from build123d import *

# Parameters (mm, degrees)
ESQUISSE1_W             = 35.1
ESQUISSE1_H             = 55.9
ESQUISSE1_W_2           = 20.1
ESQUISSE1_H_2           = 40.9
BOSS_EXTRU_1_DEPTH      = 4
ESQUISSE5_W             = 17.55
ESQUISSE5_H             = 3
BOSS_EXTRU_2_DEPTH      = 4
ESQUISSE7_W             = 11.4
ESQUISSE7_H             = 7
BOSS_EXTRU_3_DEPTH      = 6
ESQUISSE8_R             = 3
ENL_V_MAT_EXTRU_1_DEPTH = 6
CONG_1_R                = 0.5
CONG_2_R                = 0.5
ENL_V_MAT_EXTRU_2_REACH = 47.983
ESQUISSE9_R             = 2.25


with BuildPart() as part:
    # Esquisse1 → Boss.-Extru.1 (new body)
    with BuildSketch(Plane(origin=(0, 0, 0), x_dir=(1, 0, 0), z_dir=(0, 1, 0))):
        with Locations((-6.45, -0.55)):
            Rectangle(ESQUISSE1_W, ESQUISSE1_H)
        with Locations((-6.45, -0.55)):
            Rectangle(ESQUISSE1_W_2, ESQUISSE1_H_2, mode=Mode.SUBTRACT)
    extrude(amount=BOSS_EXTRU_1_DEPTH)

    # Esquisse5 → Boss.-Extru.2 (add)
    with BuildSketch(Plane.XY.offset(28.5)):
        with Locations((2.325, 5.5)):
            Rectangle(ESQUISSE5_W, ESQUISSE5_H)
    boss_extru_2 = extrude(amount=-BOSS_EXTRU_2_DEPTH)

    # Symétrie1: Boss.-Extru.2 across plane
    add(boss_extru_2.mirror(Plane(origin=(-6.45, 0, 0), x_dir=(0, 0, 1), z_dir=(1, 0, 0))))

    # Esquisse7 → Boss.-Extru.3 (add)
    with BuildSketch(Plane.XY.offset(28.5)):
        with Locations((16.8, 3.5)):
            Rectangle(ESQUISSE7_W, ESQUISSE7_H)
    boss_extru_3 = extrude(amount=-BOSS_EXTRU_3_DEPTH)

    # Esquisse8 → Enlèv. mat.-Extru.1 (cut)
    with BuildSketch(Plane(origin=(0, 0, 22.5), x_dir=(-1, 0, 0), z_dir=(0, 0, -1))):
        with Locations((-16.8, 3.5)):
            Circle(ESQUISSE8_R)
    enl_v_mat_extru_1 = extrude(amount=-ENL_V_MAT_EXTRU_1_DEPTH, mode=Mode.SUBTRACT)

    # Symétrie2: Boss.-Extru.3 across plane
    add(boss_extru_3.mirror(Plane(origin=(-6.45, 0, 0), x_dir=(0, 0, 1), z_dir=(1, 0, 0))))

    # Symétrie3: Enlèv. mat.-Extru.1 across plane
    add(enl_v_mat_extru_1.mirror(Plane(origin=(-6.45, 0, 0), x_dir=(0, 0, 1), z_dir=(1, 0, 0))), mode=Mode.SUBTRACT)

    # Congé1
    cong_1_edges = [part.edges().sort_by_distance(p)[0] for p in [
        (11.1, 7, 23.5),
        (-24, 7, 23.5),
        (-24, 0, -2.45),
        (11.1, 0, -2.45),
        (11.1, 5.5, 24.5),
        (-6.45, 7, 24.5),
        (-24, 5.5, 24.5),
        (-6.45, 4, 24.5),
        (-29.7, 7, 22.5),
        (-35.4, 3.5, 22.5),
        (-29.7, 0, 22.5),
        (-24, 2, 22.5),
        (11.1, 2, 22.5),
        (16.8, 0, 22.5),
        (22.5, 3.5, 22.5),
        (16.8, 7, 22.5),
    ]]
    fillet(cong_1_edges, radius=CONG_1_R - 0.0001)  # a hair under: the kernel refuses the full size

    # Congé2
    cong_2_edges = [part.edges().sort_by_distance(p)[0] for p in [
        (-6.45, 0, -27.4),
        (10.95358268, 0.14641732, -27.4),
        (-23.85358268, 0.14641732, -27.4),
        (-6.45, 4, -27.4),
        (11.1, 2.24995, -27.4),
        (-24, 2.24995, -27.4),
    ]]
    fillet(cong_2_edges, radius=CONG_2_R - 0.0001)  # a hair under: the kernel refuses the full size

    # Esquisse9 → Enlèv. mat.-Extru.2 (cut, up to next)
    with BuildSketch(Plane.XZ, mode=Mode.PRIVATE) as enl_v_mat_extru_2_sk1:
        with Locations(Location((-1.95, -24.9, 0), (0, 0, 297.266044451))):
            Circle(ESQUISSE9_R)
    enl_v_mat_extru_2_tool1 = extrude(enl_v_mat_extru_2_sk1.sketch, amount=-ENL_V_MAT_EXTRU_2_REACH, mode=Mode.PRIVATE) & part.part
    # Esquisse9 → Enlèv. mat.-Extru.2 (cut, up to next)
    with BuildSketch(Plane.XZ, mode=Mode.PRIVATE) as enl_v_mat_extru_2_sk2:
        with Locations(Location((-10.95, -24.9, 0), (0, 0, 242.733955549))):
            Circle(ESQUISSE9_R)
    enl_v_mat_extru_2_tool2 = extrude(enl_v_mat_extru_2_sk2.sketch, amount=-ENL_V_MAT_EXTRU_2_REACH, mode=Mode.PRIVATE) & part.part
    add(enl_v_mat_extru_2_tool1.solids().sort_by_distance((-1.95, 0, -24.9))[0], mode=Mode.SUBTRACT)
    add(enl_v_mat_extru_2_tool2.solids().sort_by_distance((-10.95, 0, -24.9))[0], mode=Mode.SUBTRACT)


solid = part.part
Geometry check sheet. Reference: the model listing, model coordinates, mm. A direction names the side the tool comes from. Give positions to 0.01 mm unless a question says otherwise; leave off trailing zeros. Write each loop counter-clockwise with the first axis right and the second up, starting at its lowest first coordinate (ties: lowest second). Pieces come first, ordered by that corner, then holes. Notation, with made-up numbers: M 83.25,-6 L 95.25,-6 A33 ccw 95.25,25 Z; hole C 43.25,84.5 d5. An arc over 180 degrees is marked long. One line per question, with ' | ' between items.
1. Set-up check for faces 1 (the face through (-7, 2, -27.4)), 2 (the face through (-32.7, 3.6, 25.5)), 3 (the face through (-7, 2, -19.9)), 4 (the face through (11.1, 2, -2)), 5 (the face through (11.1, 5, 23)): record each of +Z, -Z, +X, -X, +Y, -Y from which the full face is reachable in a straight line by a thin tool's end or side.
Ans:
face 1: -Z, +X, -X, +Y, -Y | face 2: +Z, -Z | face 3: +Y, -Y | face 4: -Z, +X, +Y, -Y | face 5: -Z, +Y
2. Cross-section at B-B (y = 2.5). Enter the section's corners in (x, z), plus the area to 3 significant figures.
Ans:
outline: M -35.4,23 A0.5 ccw -34.9,22.5 L -32.53,22.5 L -32.53,28.5 L -35.4,28.5 Z; M -26.87,22.5 L -24.5,22.5 A0.5 cw -24,22 L -24,-26.9 A0.5 ccw -23.5,-27.4 L 10.6,-27.4 A0.5 ccw 11.1,-26.9 L 11.1,22 A0.5 cw 11.6,22.5 L 13.97,22.5 L 13.97,28.5 L -26.87,28.5 Z; M 19.63,22.5 L 22,22.5 A0.5 ccw 22.5,23 L 22.5,28.5 L 19.63,28.5 Z; hole M -16.5,-19.9 L 3.6,-19.9 L 3.6,21 L -16.5,21 Z; hole C -10.95,-24.9 d4.5; hole C -1.95,-24.9 d4.5 | area: 1,180 mm2
3. Mould release check, pull along Z, two halves, no side actions. Record for faces 6 (the face through (-16.5, 2, 1)), 7 (the face through (-7, 2, 21)), 8 (the face through (14, 2, 22.5)), 9 (the face through (-6, 7, 26)): released by +Z, released by -Z, zero draft, split by the parting line, or undercut.
Ans:
face 6: undercut | face 7: undercut | face 8: released by -Z | face 9: zero draft
4. Cross-section at C-C (z = 3). Enter the section's corners in (x, y), plus the area to 3 significant figures.
Ans:
outline: M -24,0.5 A0.5 ccw -23.5,0 L -16.5,0 L -16.5,4 L -24,4 Z; M 3.6,0 L 10.6,0 A0.5 ccw 11.1,0.5 L 11.1,4 L 3.6,4 Z | area: 59.9 mm2
5. Cross-section at D-D (x = -1.95). Enter the section's corners in (y, z).
Ans:
outline: M 0,-22.65 L 4,-22.65 L 4,-19.9 L 0,-19.9 Z; M 0,21 L 4,21 L 4,24 A0.5 cw 4.5,24.5 L 6.5,24.5 A0.5 ccw 7,25 L 7,28.5 L 0,28.5 Z; M 0.07,-27.15 A0.5 ccw 0.5,-27.4 L 3.5,-27.4 A0.5 ccw 3.93,-27.15 Z
6. Scan lines: line 1 along Z through (x, y) = (-1.95, 2.1); line 2 along Y through (x, z) = (16.8, 27.15); line 3 along X through (y, z) = (2.3, -24.9). Record each from-to range of solid material in increasing order. Write a range as from..to.
Ans:
line 1: -27.4..-27.15, -22.65..-19.9, 21..28.5 | line 2: 0..0.5, 6.5..7 | line 3: -24..-13.2, -8.7..-4.2, 0.3..11.1
7. Cross-section at A-A (x = 15). Enter the section's corners in (y, z), plus the area to 3 significant figures.
Ans:
outline: M 0,23 A0.5 ccw 0.5,22.5 L 1.1,22.5 L 1.1,28.5 L 0,28.5 Z; M 5.9,22.5 L 6.5,22.5 A0.5 ccw 7,23 L 7,28.5 L 5.9,28.5 Z | area: 13.1 mm2
8. Gauge pin test, flat ends, axial feed: pin 1 (1.5 mm diameter, centred on x = -22.5, z = -12.5, fed in from +Y); pin 2 (2 mm diameter, centred on y = 3, z = -9, fed in from +X); pin 3 (1.2 mm diameter, centred on y = 3, z = 6, fed in from -X). Record the tip position at first contact, or that the pin passes through.
Ans:
pin 1: y = 4 | pin 2: x = 11.1 | pin 3: x = -24
